```python
from build123d import *

# Parameters (mm, degrees)
SKETCH1_R           = 3
BOSS_EXTRUDE1_DEPTH = 40
FILLET1_R           = 2


with BuildPart() as part:
    # Sketch1 → Boss-Extrude1 (new body)
    with BuildSketch(Plane.XY):
        with BuildLine():
            Line((-1.5, 5.809475019), (-1.5, 11))
            Line((-1.5, 11), (1.5, 11))
            Line((1.5, 11), (1.5, 5.809475019))
            ThreePointArc((1.5, 5.809475019), (0, -6), (-1.5, 5.809475019))
        make_face()
        Circle(SKETCH1_R, mode=Mode.SUBTRACT)
    extrude(amount=BOSS_EXTRUDE1_DEPTH)

    # Fillet1
    fillet1_edges = [part.edges().sort_by_distance(p)[0] for p in [
        (1.5, 5.809475019, 20),
        (-1.5, 5.809475019, 20),
    ]]
    fillet(fillet1_edges, radius=FILLET1_R)


solid = part.part
```
Here's how the part is built. I have some questions about the finished solid (model axes, mm). A direction names the side the tool comes from. Coordinates: 2 decimals unless noted, no trailing zeros. Loops run counter-clockwise (first coordinate to the right, second up) from the corner with the lowest first, then second, coordinate; pieces in that order, holes last. Notation, with made-up numbers: (11.25, 10) - (22.25, 10) arc R12 ccw to (22.25, 17) - close; hole circle Ø2 at (80.5, 55.25). An arc over 180 degrees is marked (long way). Return JSON: item names as keys, results as strings. Group by question number.
Item 1: If we section it at A-A on y = 0: Write out the boundary of the cut face in (x, z), and give its area (3 significant figures).
Item 2: I need wall thicknesses on line 1 (Y direction, x = 0, z = 16.5); line 2 (X direction, y = 2.25, z = 13.5); line 3 (Y direction, x = 2, z = 28.5). Which ranges of each line are inside material? Lowest first, please. Write a range as from..to.
Item 3: On a 3-axis mill with a long thin cutter (end or side, diameter ignored), from which of +Z, -Z, +X, -X, +Y, -Y can I reach the whole of each face in a straight line? I mean faces 1 (the face through (-3, 3, 0)), 2 (the face through (1.5, 9, 20)), 3 (the face through (-1.5, 9, 20)). Say none if no direction works.
Item 4: If we section it at B-B on x = 0: Write out the boundary of the cut face in (y, z).
Item 5: Will these pins go through, and if not, where does the flat tip stop? P1, Ø1, axis at y = -1.5, z = 8, coming from the +X side; P2, Ø1, axis at x = -2.5, z = 29, coming from the +Y side; P3, Ø1, axis at x = 1.5, z = 8.5, coming from the -Y side; P4, Ø3.5, axis at x = 0, y = 0, coming from the -Z side.
Item 6: If we section it at D-D on y = 9: Write out the boundary of the cut face in (x, z), and give its area (3 significant figures).
Item 7: If we section it at C-C on z = 34: Write out the boundary of the cut face in (x, y) (3 decimals), and give its area (3 significant figures).
Calculated:
{
 "1": {"outline": "(-6, 0) - (-3, 0) - (-3, 40) - (-6, 40) - close; (3, 0) - (6, 0) - (6, 40) - (3, 40) - close", "area": "240 mm^2"},
 "2": {"line 1": "y = -6..-3, 3..11", "line 2": "x = -5.56..-1.98, 1.98..5.56", "line 3": "y = -5.66..-2.24, 2.24..5.87"},
 "3": {"face 1": "-Z, +X, -X, +Y, -Y", "face 2": "+Z, -Z, +X, +Y", "face 3": "+Z, -Z, -X, +Y"},
 "4": {"outline": "(-6, 0) - (-3, 0) - (-3, 40) - (-6, 40) - close; (3, 0) - (11, 0) - (11, 40) - (3, 40) - close"},
 "5": {"P1": "stops at x = 5.92", "P2": "stops at y = 5.87", "P3": "stops at y = -5.92", "P4": "passes through"},
 "6": {"outline": "(-1.5, 0) - (1.5, 0) - (1.5, 40) - (-1.5, 40) - close", "area": "120 mm^2"},
 "7": {"outline": "(-2.625, 5.395) arc R6 ccw (long way) to (2.625, 5.395) arc R2 cw to (1.5, 7.194) - (1.5, 11) - (-1.5, 11) - (-1.5, 7.194) arc R2 cw to start; hole circle Ø6 at (0, 0)", "area": "101 mm^2"}
}
